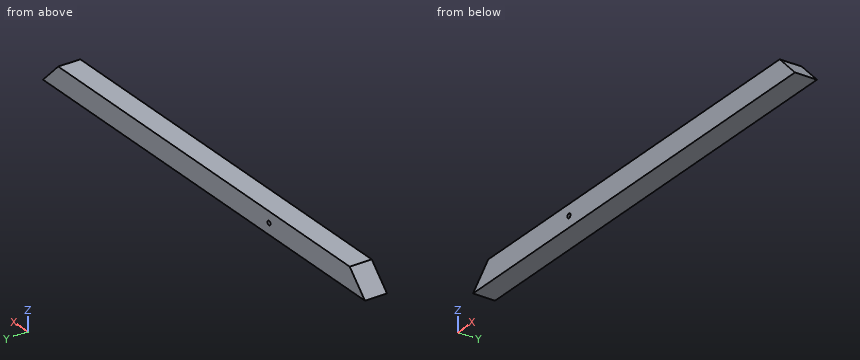
from build123d import *

# Parameters (mm, degrees)
F0_W     = 670.999928
F0_H     = 31.75
F1_DEPTH = 31.75
F3_DEPTH = 31.751
F4_R     = 3.175
F5_DEPTH = 31.751


with BuildPart() as f1:
    # F0 (on Front) → F1 (new body)
    with BuildSketch(Plane.XZ):
        Rectangle(F0_W, F0_H)
    extrude(amount=F1_DEPTH)

    # F2 (on face) → F3 (cut, through all)
    with BuildSketch(Plane.XZ.offset(31.75)):
        Polygon((-335.499964, 15.875), (-335.499964, -15.875), (-303.749964, 15.875), align=None)
        Polygon((303.749964, 15.875), (335.499964, -15.875), (335.499964, 15.875), align=None)
    extrude(amount=-F3_DEPTH, mode=Mode.SUBTRACT)

    # F4 (on face) → F5 (cut, through all)
    with BuildSketch(Plane.XZ.offset(31.75)):
        with Locations((-135.499856, 0)):
            Circle(F4_R)
    extrude(amount=-F5_DEPTH, mode=Mode.SUBTRACT)


solid = f1.part
Design review of the part built by this model. Coordinates are the model's own, in mm. Give positions to 0.01 mm unless a question says otherwise; leave off trailing zeros. Order: outer loops, then holes, each group sorted by start corner. A loop starts at its lowest first (then second) coordinate and runs counter-clockwise, first axis right, second up.
1. Add section A-A, the plane y = -10.5. State the section outline as (x, z) points (3 decimals).
Solution:
outline: (-335.5, -15.875) - (335.5, -15.875) - (303.75, 15.875) - (-303.75, 15.875) - close; hole circle Ø6.35 at (-135.5, 0)
2. For pin 1 Ø3 at (y, z) = (-23.5, 1.5) entering from -X; pin 2 Ø1 at (y, z) = (-20.5, -9) entering from -X, all flat-tipped, find the tip position at first contact; note any pin that passes through.
Solution:
pin 1: stops at x = -319.62
pin 2: stops at x = -329.12
3. To check wall thickness, follow L1, parallel to X at y = -7.5, z = 11; L2, parallel to X at y = -16, z = -13. State the ranges of each line that lie inside material, in increasing order.
Solution:
L1: x = -308.62 to 308.62
L2: x = -332.62 to 332.62
4. Add section B-B, the plane z = 11. State the section outline as (x, y) points.
Solution:
outline: (-308.62, -31.75) - (308.62, -31.75) - (308.62, 0) - (-308.62, 0) - close
